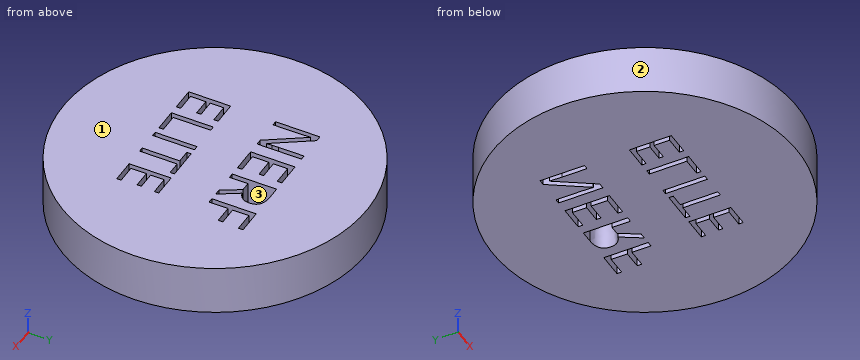
```python
from build123d import *

# Parameters (mm, degrees)
F0_R     = 76.4498287505
F0_W     = 2.4511385491
F0_H     = 21.0908701144
F1_DEPTH = 25.4


# Not quite as in the source:
# - a feature names something its author has since deleted; it is built from what else it names


with BuildPart() as f1:
    # F0 (on Top) → F1 (new body)
    with BuildSketch(Plane.XY):
        Circle(F0_R)
        with BuildLine():
            Line((-18.3724183589, -37.9301533103), (-18.3724183589, -42.5397194922))
            ThreePointArc((-18.3724183589, -42.5397194922), (-20.6772014499, -40.2349364012), (-18.3724183589, -37.9301533103))
        make_face(mode=Mode.SUBTRACT)
        Polygon((-23.2161222044, -29.6504020767), (-23.2161222044, -31.8430401385), (-34.9732782957, -31.8430401385), (-34.9732782957, -10.7521700241), (-23.2161222044, -10.7521700241), (-23.2161222044, -12.9309598455), (-32.5221397466, -12.9309598455), (-32.5221397466, -19.725829797), (-23.7792839802, -19.725829797), (-23.7792839802, -21.890771378), (-32.5221397466, -21.890771378), (-32.5221397466, -29.6504020767), align=None, mode=Mode.SUBTRACT)
        Polygon((-6.7874930214, -31.8430401385), (-18.5446491127, -31.8430401385), (-18.5446491127, -10.7521700241), (-16.0935105636, -10.7521700241), (-16.0935105636, -29.6227055959), (-6.7874930214, -29.6227055959), align=None, mode=Mode.SUBTRACT)
        with Locations((-1.984461646, -21.2976050813)):
            Rectangle(F0_W, F0_H, mode=Mode.SUBTRACT)
        Polygon((11.5152646944, -12.9309598455), (11.5152646944, -31.8430401385), (9.0641261454, -31.8430401385), (9.0641261454, -12.9309598455), (2.3846581971, -12.9309598455), (2.3846581971, -10.7521700241), (18.1947326427, -10.7521700241), (18.1947326427, -12.9309598455), align=None, mode=Mode.SUBTRACT)
        Polygon((33.1277518635, -29.6504020767), (33.1277518635, -31.8430401385), (21.3705957722, -31.8430401385), (21.3705957722, -10.7521700241), (33.1277518635, -10.7521700241), (33.1277518635, -12.9309598455), (23.8217343212, -12.9309598455), (23.8217343212, -19.725829797), (32.5645900876, -19.725829797), (32.5645900876, -21.890771378), (23.8217343212, -21.890771378), (23.8217343212, -29.6504020767), align=None, mode=Mode.SUBTRACT)
        with BuildLine():
            Line((-17.3598606786, 34.2694889666), (-17.3598606786, 11.9390692562))
            Line((-17.3598606786, 11.9390692562), (-20.321610371, 11.9390692562))
            Line((-20.321610371, 11.9390692562), (-32.5253875688, 30.677267805))
            Line((-32.5253875688, 30.677267805), (-32.647571962, 30.677267805))
            add(Edge.make_bspline(
                [(-32.647571962, 30.677267805), (-32.4032031755, 27.3782891873), (-32.4032031755, 24.631584027)],
                knots=[0, 0, 0, 1, 1, 1], degree=2))
            Line((-32.4032031755, 24.631584027), (-32.4032031755, 11.9390692562))
            Line((-32.4032031755, 11.9390692562), (-34.8029046589, 11.9390692562))
            Line((-34.8029046589, 11.9390692562), (-34.8029046589, 34.2694889666))
            Line((-34.8029046589, 34.2694889666), (-31.8704792209, 34.2694889666))
            Line((-31.8704792209, 34.2694889666), (-19.6960262775, 15.6046010537))
            Line((-19.6960262775, 15.6046010537), (-19.5738418843, 15.6046010537))
            add(Edge.make_bspline(
                [(-19.5738418843, 15.6046010537), (-19.6031661386, 16.015140615), (-19.7106884047, 18.2535586993)],
                knots=[0, 0, 0, 1, 1, 1], degree=2))
            add(Edge.make_bspline(
                [(-19.7106884047, 18.2535586993), (-19.8182106708, 20.4919767837), (-19.7888864164, 21.4547898025)],
                knots=[0, 0, 0, 1, 1, 1], degree=2))
            Line((-19.7888864164, 21.4547898025), (-19.7888864164, 34.2694889666))
            Line((-19.7888864164, 34.2694889666), (-17.3598606786, 34.2694889666))
        make_face(mode=Mode.SUBTRACT)
        Polygon((1.2268292226, 14.2605727279), (1.2268292226, 11.9390692562), (-11.2213167617, 11.9390692562), (-11.2213167617, 34.2694889666), (1.2268292226, 34.2694889666), (1.2268292226, 31.962647622), (-8.6261202491, 31.962647622), (-8.6261202491, 24.7684305474), (0.6305693836, 24.7684305474), (0.6305693836, 22.4762513301), (-8.6261202491, 22.4762513301), (-8.6261202491, 14.2605727279), align=None, mode=Mode.SUBTRACT)
        with BuildLine():
            Line((13.4306064204, 21.2250831432), (8.768049974, 21.2250831432))
            Line((8.768049974, 21.2250831432), (8.768049974, 11.9390692562))
            Line((8.768049974, 11.9390692562), (6.1728534614, 11.9390692562))
            Line((6.1728534614, 11.9390692562), (6.1728534614, 34.2694889666))
            Line((6.1728534614, 34.2694889666), (12.2967352511, 34.2694889666))
            add(Edge.make_bspline(
                [(12.2967352511, 34.2694889666), (16.40701824, 34.2694889666), (18.3692995956, 32.6957539815)],
                knots=[0, 0, 0, 1, 1, 1], degree=2))
            add(Edge.make_bspline(
                [(18.3692995956, 32.6957539815), (20.3315809512, 31.1220189964), (20.3315809512, 27.9598868991)],
                knots=[0, 0, 0, 1, 1, 1], degree=2))
            add(Edge.make_bspline(
                [(20.3315809512, 27.9598868991), (20.3315809512, 23.5319244877), (15.8400826553, 21.9728516299)],
                knots=[0, 0, 0, 1, 1, 1], degree=2))
            Line((15.8400826553, 21.9728516299), (21.9053159362, 11.9390692562))
            Line((21.9053159362, 11.9390692562), (18.8360439778, 11.9390692562))
            Line((18.8360439778, 11.9390692562), (13.4306064204, 21.2250831432))
        make_face(mode=Mode.SUBTRACT)
        Polygon((28.1025083619, 21.4841140569), (28.1025083619, 11.9390692562), (25.5073118492, 11.9390692562), (25.5073118492, 34.2694889666), (37.9554578336, 34.2694889666), (37.9554578336, 31.962647622), (28.1025083619, 31.962647622), (28.1025083619, 23.7909554014), (37.3591979945, 23.7909554014), (37.3591979945, 21.4841140569), align=None, mode=Mode.SUBTRACT)
        with BuildLine():
            ThreePointArc((-18.3724183589, -37.9301533103), (-20.6772014499, -40.2349364012), (-18.3724183589, -42.5397194922))
            Line((-18.3724183589, -42.5397194922), (-18.3724183589, -37.9301533103))
        make_face()
    extrude(amount=F1_DEPTH)


solid = f1.part
```
Source: CAD feature listing. Evaluate the final solid. Frame: model axes, mm. Face numbers are marked on the shaded views. Give positions to 0.01 mm unless a question says otherwise; leave off trailing zeros. Loops run counter-clockwise (first coordinate to the right, second up) from the corner with the lowest first, then second, coordinate; pieces in that order, holes last. Notation, with made-up numbers: (-3, 57.5) - (17, 57.5) arc R19 ccw to (17, 93.5) - close; hole circle Ø8 at (46.5, 77.5). An arc over 180 degrees is marked (long way). Use CSV: the item, a comma, the result in double quotes. Start each with the question number.
1. Ray query, L1, parallel to Y at x = -2, z = 6.75; L2, parallel to Y at x = 14.5, z = 5.5; L3, parallel to X at y = -19.5, z = 4.75. Return the intervals inside material, ascending.
2. Draft query along X for the marked faces 1, 2 and 3. Return one class per face: +X half, -X half, draft (parallel to the pull), parting line (faces both ways), or undercut.
3. Section A-A (z = 5). Count the separate pieces of the cut face and the enclosed holes in it, then the cut area to 3 significant figures.
4. Section C-C (x = 48.5). Output: boundary loops of the cut face in (y, z), then the cut area to 3 significant figures.
5. Pin query (flat end, axial travel): pin 1 (8 mm diameter, centred on y = -57.5, z = 19.5, fed in from -X); pin 2 (4.5 mm diameter, centred on x = 28, z = 8, fed in from -Y); pin 3 (0.7 mm diameter, centred on y = -11.5, z = 12, fed in from +X). Return the tip coordinate at first contact, or that it passes through.
6. Section D-D (x = -56.5). Output: boundary loops of the cut face in (y, z).
Response:
1,L1,"-76.42 to -31.84, -10.75 to 11.94, 14.26 to 22.48, 24.77 to 31.96, 34.27 to 76.42"
1,L2,"-75.06 to -12.93, -10.75 to 19.39, 34.14 to 75.06"
1,L3,"-73.92 to -34.97, -32.52 to -18.54, -16.09 to -3.21, -0.76 to 9.06, 11.52 to 21.37, 23.82 to 73.92"
2,face 1,"draft"
2,face 2,"parting line"
2,face 3,"undercut"
3,separate pieces,"1"
3,enclosed holes,"9"
3,area,"17,300 mm²"
4,outline,"(-59.1, 0) - (59.1, 0) - (59.1, 25.4) - (-59.1, 25.4) - close"
4,area,"3,000 mm²"
5,pin 1,"x = -54.61"
5,pin 2,"y = -71.98"
5,pin 3,"x = 75.63"
6,outline,"(-51.5, 0) - (51.5, 0) - (51.5, 25.4) - (-51.5, 25.4) - close"
